```python
from build123d import *

# Parameters (mm, degrees)
ESBO_O1_W                = 60
ESBO_O1_H                = 12
RESSALTO_EXTRUS_O1_DEPTH = 4
ESBO_O3_W                = 25
ESBO_O3_H                = 12
CORTE_EXTRUS_O2_DEPTH    = 10
ESBO_O4_W                = 5
ESBO_O4_H                = 12
RESSALTO_EXTRUS_O2_DEPTH = 4
CORTE_EXTRUS_O3_DEPTH    = 41.644802866
ESBO_O6_W                = 40
ESBO_O6_H                = 7
RESSALTO_EXTRUS_O3_DEPTH = 1
ESBO_O2_R                = 2
CORTE_EXTRUS_O1_DEPTH    = 15
ESBO_O7_W                = 2.5
ESBO_O7_H                = 1
RESSALTO_EXTRUS_O4_DEPTH = 40


with BuildPart() as part:
    # Esboço1 → Ressalto-extrusão1 (new body)
    with BuildSketch(Plane(origin=(0, 0, 0), x_dir=(0, 0, -1), z_dir=(1, 0, 0))):
        Rectangle(ESBO_O1_W, ESBO_O1_H)
    extrude(amount=RESSALTO_EXTRUS_O1_DEPTH)

    # Esboço3 → Corte-extrusão2 (cut)
    with BuildSketch(Plane.ZY):
        with Locations((17.5, 0)):
            Rectangle(ESBO_O3_W, ESBO_O3_H)
    extrude(amount=-CORTE_EXTRUS_O2_DEPTH, mode=Mode.SUBTRACT)

    # Esboço4 → Ressalto-extrusão2 (add)
    with BuildSketch(Plane.ZY):
        with Locations((-32.5, 0)):
            Rectangle(ESBO_O4_W, ESBO_O4_H)
    extrude(amount=-RESSALTO_EXTRUS_O2_DEPTH)

    # Esboço5 → Corte-extrusão3 (cut, through all)
    with BuildSketch(Plane.XY.offset(5)):
        Polygon((4, 6), (2.5, 6), (4, 4.5), align=None)
        Polygon((4, -4.5), (4, -6), (2.5, -6), align=None)
    extrude(amount=-CORTE_EXTRUS_O3_DEPTH, mode=Mode.SUBTRACT)

    # Esboço6 → Ressalto-extrusão3 (add)
    with BuildSketch(Plane(origin=(4, 0, 0), x_dir=(0, 0, -1), z_dir=(1, 0, 0))):
        with Locations((15, 0)):
            Rectangle(ESBO_O6_W, ESBO_O6_H)
    extrude(amount=RESSALTO_EXTRUS_O3_DEPTH)

    # Esboço2 → Corte-extrusão1 (cut)
    with BuildSketch(Plane.ZY):
        with Locations((-20, 0)):
            Circle(ESBO_O2_R)
        with Locations((-10, 0)):
            Circle(ESBO_O2_R)
    extrude(amount=-CORTE_EXTRUS_O1_DEPTH, mode=Mode.SUBTRACT)

    # Esboço7 → Ressalto-extrusão4 (add)
    with BuildSketch(Plane(origin=(0, 0, -35), x_dir=(-1, 0, 0), z_dir=(0, 0, -1))):
        with Locations((-1.25, 6.5)):
            Rectangle(ESBO_O7_W, ESBO_O7_H)
        with Locations((-1.25, -6.5)):
            Rectangle(ESBO_O7_W, ESBO_O7_H)
    extrude(amount=-RESSALTO_EXTRUS_O4_DEPTH)


solid = part.part
```
Design review of the part built by this model. Coordinates are the model's own, in mm. A direction names the side the tool comes from. Give positions to 0.01 mm unless a question says otherwise; leave off trailing zeros. Loops run counter-clockwise (first coordinate to the right, second up) from the corner with the lowest first, then second, coordinate; pieces in that order, holes last. Notation, with made-up numbers: M -6.5,27.25 L 36.5,27.25 A19 ccw 36.5,58.25 Z; hole C -16,32.25 d5. An arc over 180 degrees is marked long. Return JSON: item names as keys, results as strings. Group by question number.
Item 1: Mouldability with a two-part tool opening along Y and no side actions: class faces 1 (the flat face through (4.5, -3.5, -14.7)), 2 (the flat face through (4, -4, -15)), 3 (the cylindrical face through (2.5, -1.2, -21.6)) as released by +Y, released by -Y, zero draft, split by the parting line, or undercut.
Item 2: Insertion check: pin 1 Ø0.5 at (y, z) = (-4, -6.5) entering from +X; pin 2 Ø3 at (y, z) = (0, -20) entering from +X; pin 3 Ø1.5 at (x, z) = (4, -7) entering from +Y; pin 4 Ø0.8 at (y, z) = (6.5, -14) entering from +X. Each pin has a flat end and moves straight along its axis. Give the tip position at first contact, or say it passes through.
Item 3: We need section B-B (y = 0). Give the boundary of the cut face in (x, z), and give its area (3 significant figures).
Item 4: We need section A-A (z = -10). Give the boundary of the cut face in (x, y).
Item 5: Tool access review of faces 4 (the flat face through (4.5, 3.5, -14.7)), 5 (the flat face through (2.5, -6.5, -15.3)), 6 (the flat face through (2, 0, -35)): name each direction out of +Z, -Z, +X, -X, +Y, -Y from which nothing blocks a thin tool from reaching the whole face with its end or side.
Item 6: We need section D-D (z = -24). Give the boundary of the cut face in (x, y), and give its area (4 significant figures).
Item 7: For probe 1 along Z at (x, y) = (3.95, 1.5); probe 2 along Y at (x, z) = (1.1, -20); probe 3 along Z at (x, y) = (1.4, 1.25), list the stretches that pass through material, from the lowest coordinate up.
Item 8: We need section C-C (x = 0.6). Give the boundary of the cut face in (y, z), and give its area (3 significant figures).
Output:
{
 "1": {"face 1": "released by -Y", "face 2": "zero draft", "face 3": "undercut"},
 "2": {"pin 1": "stops at x = 4", "pin 2": "passes through", "pin 3": "stops at y = 5.25", "pin 4": "stops at x = 2.5"},
 "3": {"outline": "M 0,-35 L 5,-35 L 5,-22 L 0,-22 Z; M 0,-18 L 5,-18 L 5,-12 L 0,-12 Z; M 0,-8 L 5,-8 L 5,5 L 0,5 Z", "area": "160 mm^2"},
 "4": {"outline": "M 0,-7 L 2.5,-7 L 2.5,-6 L 4,-4.5 L 4,-3.5 L 5,-3.5 L 5,-2 L 0,-2 Z; M 0,2 L 5,2 L 5,3.5 L 4,3.5 L 4,4.5 L 2.5,6 L 2.5,7 L 0,7 Z"},
 "5": {"face 4": "+Z, -Z, +X, +Y", "face 5": "+Z, -Z, +X, -Y", "face 6": "-Z, +X, -X, +Y, -Y"},
 "6": {"outline": "M 0,-7 L 2.5,-7 L 2.5,-6 L 4,-4.5 L 4,-3.5 L 5,-3.5 L 5,3.5 L 4,3.5 L 4,4.5 L 2.5,6 L 2.5,7 L 0,7 Z", "area": "57.75 mm^2"},
 "7": {"probe 1": "z = -35 to -21.32, -18.68 to -11.32, -8.68 to 5", "probe 2": "y = -7 to -2, 2 to 7", "probe 3": "z = -35 to -21.56, -18.44 to -11.56, -8.44 to 5"},
 "8": {"outline": "M -7,-35 L 7,-35 L 7,5 L -7,5 Z; hole C 0,-20 d4; hole C 0,-10 d4", "area": "535 mm^2"}
}
